from build123d import *

# Parameters (mm, degrees)
BOSS_EXTRUDE1_DEPTH = 38.1
SKETCH2_R           = 3.175
CUT_EXTRUDE1_DEPTH  = 39.1


with BuildPart() as part:
    # Sketch1 → Boss-Extrude1 (new body)
    with BuildSketch(Plane(origin=(0, 0, 0), x_dir=(0, 0, -1), z_dir=(1, 0, 0))):
        Polygon((6.35, -1.3864e-05), (3.175012007, 5.499254382), (-3.174987993, 5.499268246), (-6.35, 1.3864e-05), (-3.175012007, -5.499254382), (3.174987993, -5.499268246), align=None)
    extrude(amount=BOSS_EXTRUDE1_DEPTH)

    # Sketch2 → Cut-Extrude1 (cut, through all)
    with BuildSketch(Plane.ZY):
        Circle(SKETCH2_R)
    extrude(amount=-CUT_EXTRUDE1_DEPTH, mode=Mode.SUBTRACT)


solid = part.part
Here's how the part is built. I have some questions about the finished solid (model axes, mm). Coordinates: 2 decimals unless noted, no trailing zeros. Write each loop counter-clockwise with the first axis right and the second up, starting at its lowest first coordinate (ties: lowest second). Pieces come first, ordered by that corner, then holes.
1) If I drill on line 1 (Y direction, x = 19.5, z = 0) (3 decimals); line 2 (Z direction, x = 8, y = 1.75); line 3 (Z direction, x = 29.5, y = -1.5), over which ranges is the centre line in solid material (lowest first)?
Filled in:
line 1: y = -5.499 to -3.175, 3.175 to 5.499
line 2: z = -5.34 to -2.65, 2.65 to 5.34
line 3: z = -5.48 to -2.8, 2.8 to 5.48
2) Thinking about a two-plate mould opening in Y: for faces 1 (the face through (18.78, -3.1, -0.69)), 2 (the face through (18.78, 2.79, 4.74)), 3 (the face through (38.1, 3, -3)), which applies, +Y half, -Y half, draft (parallel to the pull), parting line (faces both ways), or undercut?
Filled in:
face 1: undercut
face 2: +Y half
face 3: draft
3) I'm going to push flat-ended pins straight in: pin 1 (1.5 mm diameter, centred on x = 10.5, y = -2, fed in from -Z); pin 2 (2 mm diameter, centred on x = 7, y = 2, fed in from +Z). Where does each tip first touch, or does it pass through?
Filled in:
pin 1: stops at z = -5.63
pin 2: stops at z = 5.77
4) If we section it at D-D (z = -5): List the corners of the cut face in (x, y) for me, plus the area to 3 significant figures.
Filled in:
outline: (0, -2.34) - (38.1, -2.34) - (38.1, 2.34) - (0, 2.34) - close
area: 178 mm2
5) If we section it at C-C (x = 23): List the corners of the cut face in (y, z) for me (3 decimals), plus the area to 3 significant figures.
Filled in:
outline: (-5.499, -3.175) - (0, -6.35) - (5.499, -3.175) - (5.499, 3.175) - (0, 6.35) - (-5.499, 3.175) - close; hole circle Ø6.35 at (0, 0)
area: 73.1 mm2
6) If we section it at A-A (z = 0): List the corners of the cut face in (x, y) for me (3 decimals), plus the area to 3 significant figures.
Filled in:
outline: (0, -5.499) - (38.1, -5.499) - (38.1, -3.175) - (0, -3.175) - close; (0, 3.175) - (38.1, 3.175) - (38.1, 5.499) - (0, 5.499) - close
area: 177 mm2
7) If we section it at B-B (y = 1): List the corners of the cut face in (x, z) for me.
Filled in:
outline: (0, -5.77) - (38.1, -5.77) - (38.1, -3.01) - (0, -3.01) - close; (0, 3.01) - (38.1, 3.01) - (38.1, 5.77) - (0, 5.77) - close
